Part print with two shaded views. Sizes in mm from the minimum x, y, z corner. A direction names the side the tool comes from. Coordinates: 2 decimals unless noted, no trailing zeros. Loops run counter-clockwise (first coordinate to the right, second up) from the corner with the lowest first, then second, coordinate; pieces in that order, holes last.
Item 1: 3-axis set-ups, long thin cutter, end or side, ignore diameter. For the marked faces 1 and 2: which of +Z, -Z, +X, -X, +Y, -Y reach the whole face in a straight line?
Item 2: Flat gauge pins, fed straight in: pin 1 (1 mm diameter, centred on x = 18.5, z = 14.5, fed in from +Y); pin 2 (1.5 mm diameter, centred on x = 40, y = 2, fed in from +Z); pin 3 (0.6 mm diameter, centred on y = 2.5, z = 40.5, fed in from +X). Where does each tip first touch, or does it go through?
Item 3: Cut at B-B (y = 2.7). List the corners of the cut face in (x, z).
Item 4: Cut at A-A (z = 23). List the corners of the cut face in (x, y) (3 decimals), and give its area (3 significant figures).
Item 5: Cut at C-C (x = 12). List the corners of the cut face in (y, z), and give its area (3 significant figures).
Item 6: Drill centre lines: line 1 along X through (y, z) = (1.7, 18.5); line 2 along Y through (x, z) = (11.5, 26); line 3 along Y through (x, z) = (56.5, 32). Where is each one in solid material? Low to high.
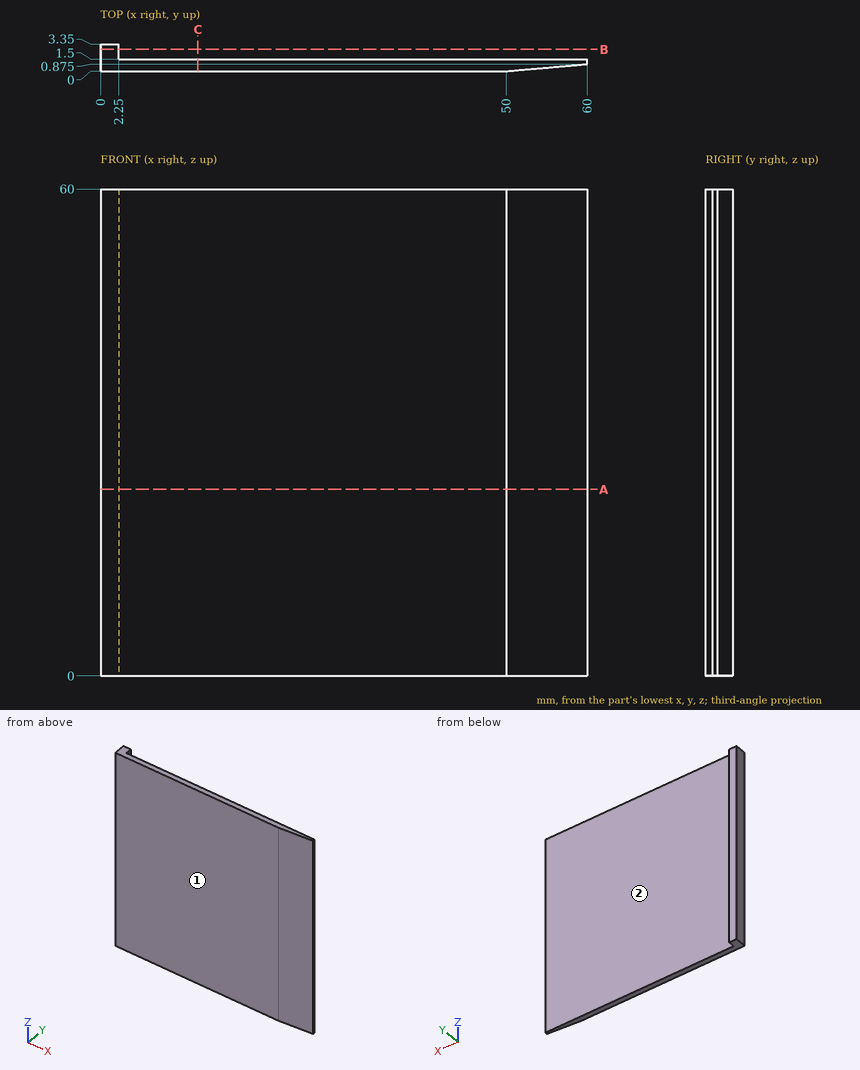
Filled sheet:
1. face 1: +Z, -Z, +X, -X, -Y
1. face 2: +Z, -Z, +X, +Y
2. pin 1: stops at y = 1.5
2. pin 2: stops at z = 60
2. pin 3: stops at x = 2.25
3. outline: (0, 0) - (2.25, 0) - (2.25, 60) - (0, 60) - close
4. outline: (0, 0) - (50, 0) - (60, 0.875) - (60, 1.5) - (2.25, 1.5) - (2.25, 3.35) - (0, 3.35) - close
4. area: 89.8 mm2
5. outline: (0, 0) - (1.5, 0) - (1.5, 60) - (0, 60) - close
5. area: 90.0 mm2
6. line 1: x = 0 to 2.25
6. line 2: y = 0 to 1.5
6. line 3: y = 0.57 to 1.5
